The listing builds one solid part. Answer for the finished solid, in the listing's coordinates (mm). Face numbers are marked on the shaded views. A direction names the side the tool comes from. Round coordinates to 2 decimals unless told otherwise and drop trailing zeros. Order: outer loops, then holes, each group sorted by start corner. A loop starts at its lowest first (then second) coordinate and runs counter-clockwise, first axis right, second up. Notation, with made-up numbers: M -34.5,6 L -7.5,6 A27 cw -7.5,26 Z; hole C 20.25,64.5 d8. An arc over 180 degrees is marked long. Write item = value, one per line. Start each with the question number.
(1) A cutting plane is placed at D-D, the plane x = 21. Determine the outline of the cut face in (y, z).
(2) Straight lines are drawn through the part: probe 1 along Y at (x, z) = (-41, 7); probe 2 along X at (y, z) = (4.5, 7); probe 3 along X at (y, z) = (7.25, 2.25). For each, find the intervals that lie inside material, in ascending order. Write a range as from..to.
(3) Which of the six approach directions +Z, -Z, +X, -X, +Y, -Y give full straight-line access (tool end or side, diameter ignored) to the marked faces 1, 2, 3 and 4?
(4) A cutting plane is placed at B-B, the plane y = -9. Determine the outline of the cut face in (x, z), and give its area (3 significant figures).
(5) A cutting plane is placed at C-C, the plane y = 8.25. Determine the outline of the cut face in (x, z).
(6) A cutting plane is placed at A-A, the plane z = 6.5. Determine the outline of the cut face in (x, y) (3 decimals), and give its area (3 significant figures).
(7) Each of these flat-tipped pins is pushed along its axis until it touches: pin 1 (2 mm diameter, centred on x = -55, z = 4, fed in from -Y); pin 2 (4 mm diameter, centred on x = 36, z = 5.5, fed in from -Y); pin 3 (4 mm diameter, centred on y = 4, z = 1.5, fed in from -X). Where does it stop, or does it pass through?
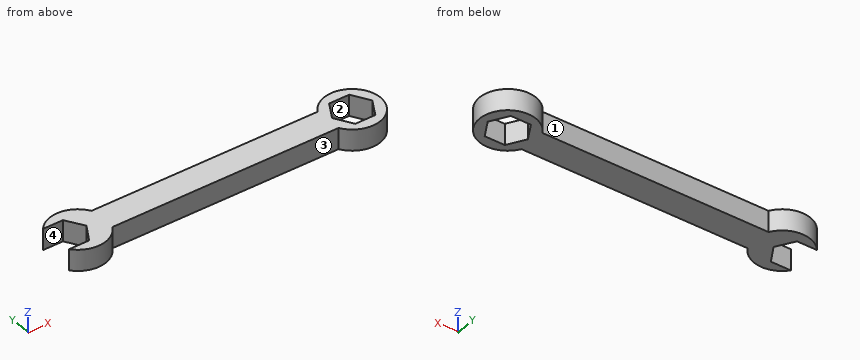
from build123d import *

# Parameters (mm, degrees)
BOSS_EXTRUDE1_DEPTH = 7.62


with BuildPart() as part:
    # Sketch1 → Boss-Extrude1 (new body)
    with BuildSketch(Plane.XY):
        with BuildLine():
            Line((-58.00496556, 6.35), (-50.723882736, 6.35))
            Line((-50.723882736, 6.35), (-46.913882736, 0))
            Line((-46.913882736, 0), (-50.723882736, -6.35))
            Line((-50.723882736, -6.35), (-58.00496556, -6.35))
            ThreePointArc((-58.00496556, -6.35), (-49.304767983, -10.130851984), (-41.275, -5.08))
            Line((-41.275, -5.08), (41.275, -5.08))
            ThreePointArc((41.275, -5.08), (60.233818102, 0), (41.275, 5.08))
            Line((41.275, 5.08), (-41.275, 5.08))
            ThreePointArc((-41.275, 5.08), (-49.304767983, 10.130851984), (-58.00496556, 6.35))
        make_face()
        Polygon((57.406166521, 0), (53.739992312, 6.35), (46.407643893, 6.35), (42.741469684, 0), (46.407643893, -6.35), (53.739992312, -6.35), align=None, mode=Mode.SUBTRACT)
    extrude(amount=BOSS_EXTRUDE1_DEPTH)


solid = part.part
Reported:
q1.outline = M -5.08,0 L 5.08,0 L 5.08,7.62 L -5.08,7.62 Z
q2.probe_1 = -5.08..5.08
q2.probe_2 = -49.61..45.34, 54.81..59.18
q2.probe_3 = -57.19..-42.96, 42.96..57.19
q3.face_1 = +Z, -Z, +Y
q3.face_2 = +Z, -Z
q3.face_3 = +Z, -Z, -Y
q3.face_4 = +Z, -Z, -X
q4.outline = M -54.79,0 L -45.36,0 L -45.36,7.62 L -54.79,7.62 Z; M 45.36,0 L 54.79,0 L 54.79,7.62 L 45.36,7.62 Z
q4.area = 144 mm²
q5.outline = M -56,0 L -44.14,0 L -44.14,7.62 L -56,7.62 Z; M 44.14,0 L 56,0 L 56,7.62 L 44.14,7.62 Z
q6.outline = M -58.005,-6.35 A10.16 ccw -41.275,-5.08 L 41.275,-5.08 A10.16 ccw long 41.275,5.08 L -41.275,5.08 A10.16 ccw -58.005,6.35 L -50.724,6.35 L -46.914,0 L -50.724,-6.35 Z; hole M 42.741,0 L 46.408,-6.35 L 53.74,-6.35 L 57.406,0 L 53.74,6.35 L 46.408,6.35 Z
q6.area = 1,190 mm²
q7.pin_1 = -9.37
q7.pin_2 = -5.08
q7.pin_3 = -50.51
